Input: part model. Units: mm. Frame: model coordinates. Face numbers are marked on the shaded views. A direction names the side the tool comes from. Coordinates: 2 decimals unless noted, no trailing zeros. Write each loop counter-clockwise with the first axis right and the second up, starting at its lowest first coordinate (ties: lowest second). Pieces come first, ordered by that corner, then holes.
1) Draft query along Z for the marked faces 1, 2, 3 and 4. Return one class per face: pulls with the +Z half, pulls with the -Z half, needs draft (parallel to the pull), parting line crosses it, or undercut.
2) Section query D-D (z = 4.5). Output: boundary loops of the cut face in (x, y), then the cut area to 3 significant figures.
3) Section query C-C (z = 10). Output: boundary loops of the cut face in (x, y).
4) Section query B-B (x = 7). Output: boundary loops of the cut face in (y, z).
5) Line query: L1, parallel to X at y = 2.1, z = 10; L2, parallel to Y at x = 33.9, z = 10; L3, parallel to Z at x = 7, y = 3.2. Output: solid intervals per line, ascending.
6) Set-up query: the marked faces 5 and 6. Return all of +Z, -Z, +X, -X, +Y, -Y with unobstructed straight access to the full face (end or side cutting, diameter ignored); none if empty.
7) Section query A-A (y = 15). Output: boundary loops of the cut face in (x, z).
8) Pin query (flat end, axial travel): pin 1 Ø5 at (x, z) = (4, 9.5) entering from +Y; pin 2 Ø6 at (x, y) = (25.5, 15.5) entering from -Z; pin 3 Ø5.5 at (y, z) = (14.5, 7.5) entering from -X. Return the tip coordinate at first contact, or that it passes through.
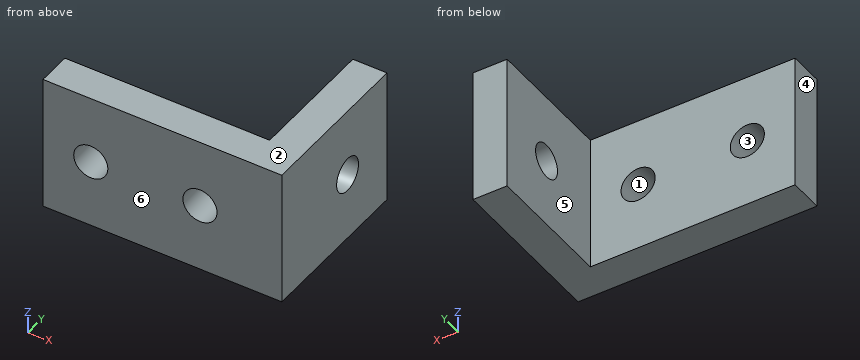
Autodesk Inventor part; units mm, degrees
ref_plane "YZ Plane" through (0, 0, 0) normal (1, 0, 0) x (0, 1, 0)
ref_plane "XZ Plane" through (0, 0, 0) normal (0, 1, 0) x (-1, 0, 0)
ref_plane "XY Plane" through (0, 0, 0) normal (0, 0, 1) x (1, 0, 0)
sketch "Sketch1" plane through (0, 0, 0) normal (0, 0, 1) x (1, 0, 0)
  line L0 (0, 0) -> (35, 0)
  line L1 (35, 0) -> (35, 5)
  line L2 (35, 5) -> (0, 5)
  line L3 (0, 5) -> (0, 0)
  line L4 (35, 5) -> (30, 5)
  line L5 (30, 5) -> (30, 24)
  line L6 (30, 24) -> (35, 24)
  line L7 (35, 24) -> (35, 5)
  dimension "d0" = 5
  dimension "d1" = 5
  dimension "d2" = 35
  dimension "d3" = 19
extrude "Extrusion1" add sketch "Sketch1" along normal blind 20
sketch "Sketch2" plane through (0, 5, 0) normal (0, 1, 0) x (1, 0, 0)
  line L0 (0, 0) -> (35, 0)
  line L1 (0, 0) -> (0, -20)
  line L2 (30, 0) -> (30, -20)
  point P0 (7, -10)
  point P1 (23, -10)
  dimension "d6" = 10
  dimension "d7" = 7
  dimension "d8" = 7
hole "Hole1" at (7, 5, 10) at (23, 5, 10) direction (0, -1, 0) diameter 5 depth 8 tip angle 118
sketch "Sketch3" plane through (30, 5, 0) normal (-1, 0, 0) x (0, 0, 1)
  line L0 (0, 19) -> (20, 19)
  line L1 (0, -5) -> (0, 19)
  line L2 (7.5, 0) -> (12.5, 0)
  line L3 (20, 19) -> (20, 0)
  point P0 (10, 10)
  dimension "d18" = 10
  dimension "d19" = 10
hole "Hole2" at (30, 15, 10) direction (1, 0, 0) diameter 5 depth 8 tip angle 118
properties part number "corner bracket"
Answer:
1. face 1: undercut
1. face 2: pulls with the +Z half
1. face 3: undercut
1. face 4: needs draft
2. outline: (0, 0) - (35, 0) - (35, 24) - (30, 24) - (30, 5) - (0, 5) - close
2. area: 270 mm2
3. outline: (0, 0) - (4.5, 0) - (4.5, 5) - (0, 5) - close; (9.5, 0) - (20.5, 0) - (20.5, 5) - (9.5, 5) - close; (25.5, 0) - (35, 0) - (35, 12.5) - (30, 12.5) - (30, 5) - (25.5, 5) - close; (30, 17.5) - (35, 17.5) - (35, 24) - (30, 24) - close
4. outline: (0, 0) - (5, 0) - (5, 7.5) - (0, 7.5) - close; (0, 12.5) - (5, 12.5) - (5, 20) - (0, 20) - close
5. L1: x = 0 to 4.5, 9.5 to 20.5, 25.5 to 35
5. L2: y = 0 to 12.5, 17.5 to 24
5. L3: z = 0 to 7.5, 12.5 to 20
6. face 5: +Z, -Z, -X, +Y
6. face 6: +Z, -Z, +X, -X, -Y
7. outline: (30, 0) - (35, 0) - (35, 7.5) - (30, 7.5) - close; (30, 12.5) - (35, 12.5) - (35, 20) - (30, 20) - close
8. pin 1: stops at y = 5
8. pin 2: passes through
8. pin 3: stops at x = 30
